```python
from build123d import *

# Parameters (mm, degrees)
RESSALTO_EXTRUS_O1_DEPTH                   = 8
BROCA_DE_ROSQUEAR_PARA_TARRAXA_DE_M6X1_0_D = 5
RESSALTO_EXTRUS_O2_DEPTH                   = 30
ESBO_O6_W                                  = 10
ESBO_O6_H                                  = 40
ESBO_O6_H_2                                = 25
CORTE_EXTRUS_O2_DEPTH                      = 20
ESBO_O14_R                                 = 3
CORTE_EXTRUS_O6_DEPTH                      = 39
ESBO_O15_R                                 = 4.25
CORTE_EXTRUS_O7_DEPTH                      = 40
RESSALTO_EXTRUS_O3_DEPTH                   = 10
ESBO_O17_W                                 = 60
ESBO_O17_H                                 = 9.5
RESSALTO_EXTRUS_O4_DEPTH                   = 30
ESBO_O18_W                                 = 9.5
ESBO_O18_H                                 = 40
RESSALTO_EXTRUS_O5_DEPTH                   = 30
FILETE1_R                                  = 5
ESBO_O19_R                                 = 2.5
CORTE_EXTRUS_O8_DEPTH                      = 10
ESBO_O20_R                                 = 2.5
CORTE_EXTRUS_O9_DEPTH                      = 10


with BuildPart() as part:
    # Esboço1 → Ressalto-extrusão1 (new body)
    with BuildSketch(Plane.XY):
        with BuildLine():
            Line((440, 72.212171493), (380, 72.212171493))
            Line((380, 72.212171493), (380, 132.212171493))
            ThreePointArc((380, 132.212171493), (382.928932188, 139.283239304), (390, 142.212171493))
            Line((390, 142.212171493), (470, 142.212171493))
            Line((470, 142.212171493), (470, 102.212171493))
            Line((470, 102.212171493), (440, 102.212171493))
            Line((440, 102.212171493), (440, 72.212171493))
        make_face()
    extrude(amount=RESSALTO_EXTRUS_O1_DEPTH)

    # Broca de rosquear para tarraxa de M6x1.01 (through all)
    with Locations(Plane.XY.offset(8)):
        with Locations((393, 87.212171493), (427, 87.212171493), (455, 112.212171493), (455, 132.212171493)):
            Hole(BROCA_DE_ROSQUEAR_PARA_TARRAXA_DE_M6X1_0_D / 2)

    # Esboço4 → Ressalto-extrusão2 (add)
    with BuildSketch(Plane(origin=(0, 0, 0), x_dir=(-1, 0, 0), z_dir=(0, 0, -1))):
        with BuildLine():
            Line((-390, 142.212171493), (-440, 142.212171493))
            Line((-440, 142.212171493), (-440, 102.212171493))
            Line((-440, 102.212171493), (-380, 102.212171493))
            Line((-380, 102.212171493), (-380, 132.212171493))
            ThreePointArc((-380, 132.212171493), (-382.928932188, 139.283239304), (-390, 142.212171493))
        make_face()
    extrude(amount=RESSALTO_EXTRUS_O2_DEPTH)

    # Esboço6 → Corte-extrusão2 (cut)
    with BuildSketch(Plane.ZY.offset(-380)):
        with Locations((-22.874860756, 122.212171493)):
            Rectangle(ESBO_O6_W, ESBO_O6_H)
        with Locations((-8.874860756, 129.712171493)):
            Rectangle(ESBO_O6_W, ESBO_O6_H_2)
    extrude(amount=-CORTE_EXTRUS_O2_DEPTH, mode=Mode.SUBTRACT)

    # Esboço14 → Corte-extrusão6 (cut, through all)
    with BuildSketch(Plane(origin=(0, 0, -30), x_dir=(-1, 0, 0), z_dir=(0, 0, -1))):
        with Locations((-390, 129.712171493)):
            Circle(ESBO_O14_R)
        with Locations((-390, 114.712171493)):
            Circle(ESBO_O14_R)
    extrude(amount=-CORTE_EXTRUS_O6_DEPTH, mode=Mode.SUBTRACT)

    # Esboço15 → Corte-extrusão7 (cut)
    with BuildSketch(Plane(origin=(0, 142.212171493, 0), x_dir=(1, 0, 0), z_dir=(0, 1, 0))):
        with Locations((420, 18.90241208)):
            Circle(ESBO_O15_R)
        with Locations((420, 1.90241208)):
            Circle(ESBO_O15_R)
    extrude(amount=-CORTE_EXTRUS_O7_DEPTH, mode=Mode.SUBTRACT)

    # Esboço16 → Ressalto-extrusão3 (add)
    with BuildSketch(Plane(origin=(0, 0, -30), x_dir=(-1, 0, 0), z_dir=(0, 0, -1))):
        with BuildLine():
            Line((-380, 102.212171493), (-440, 102.212171493))
            Line((-440, 102.212171493), (-440, 110.212171493))
            Line((-440, 110.212171493), (-440, 142.212171493))
            Line((-440, 142.212171493), (-432, 142.212171493))
            Line((-432, 142.212171493), (-432, 110.212171493))
            Line((-432, 110.212171493), (-394.815024021, 110.212171493))
            ThreePointArc((-394.815024021, 110.212171493), (-391.180367629, 108.706647521), (-387.545711238, 110.212171493))
            Line((-387.545711238, 110.212171493), (-380, 110.212171493))
            Line((-380, 110.212171493), (-380, 102.212171493))
        make_face()
    extrude(amount=RESSALTO_EXTRUS_O3_DEPTH)

    # Esboço17 → Ressalto-extrusão4 (add, through all)
    with BuildSketch(Plane.XZ.offset(-102.212171493)):
        with Locations((410, -35.25)):
            Rectangle(ESBO_O17_W, ESBO_O17_H)
    extrude(amount=RESSALTO_EXTRUS_O4_DEPTH)

    # Esboço18 → Ressalto-extrusão5 (add, through all)
    with BuildSketch(Plane(origin=(440, 0, 0), x_dir=(0, 0, -1), z_dir=(1, 0, 0))):
        with Locations((35.25, 122.212171493)):
            Rectangle(ESBO_O18_W, ESBO_O18_H)
    extrude(amount=RESSALTO_EXTRUS_O5_DEPTH)

    # Filete1
    filete1_edges = [part.edges().sort_by_distance(p)[0] for p in [
        (432, 110.212171493, -35),
    ]]
    fillet(filete1_edges, radius=FILETE1_R)

    # Esboço19 → Corte-extrusão8 (cut)
    with BuildSketch(Plane.XY.offset(-30.5)):
        with Locations((455, 132.212171493)):
            Circle(ESBO_O19_R)
        with Locations((455, 112.212171493)):
            Circle(ESBO_O19_R)
    extrude(amount=-CORTE_EXTRUS_O8_DEPTH, mode=Mode.SUBTRACT)

    # Esboço20 → Corte-extrusão9 (cut)
    with BuildSketch(Plane.XY.offset(-30.5)):
        with Locations((427, 87.212171493)):
            Circle(ESBO_O20_R)
        with Locations((393, 87.212171493)):
            Circle(ESBO_O20_R)
    extrude(amount=-CORTE_EXTRUS_O9_DEPTH, mode=Mode.SUBTRACT)


solid = part.part
```
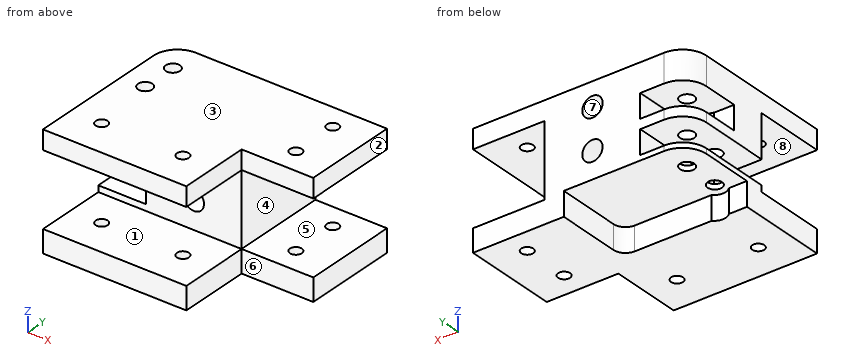
Could you check a few things on this model? Use its own coordinates, in mm. Face numbers are marked on the shaded views. A direction names the side the tool comes from. Give positions to 0.01 mm unless a question says otherwise; leave off trailing zeros. Order: outer loops, then holes, each group sorted by start corner. A loop starts at its lowest first (then second) coordinate and runs counter-clockwise, first axis right, second up.
Q1. Suppose I cut it at C-C, the plane z = -11. Write out the boundary of the cut face in (x, y).
Q2. Suppose I cut it at D-D, the plane x = 455. Write out the boundary of the cut face in (y, z).
Q3. Suppose I cut it at B-B, the plane y = 92.5. Write out the boundary of the cut face in (x, z).
Q4. We'd pull the mould along Z, two halves only. Please class the marked faces 1, 2, 3 and 4: +Z half, -Z half, draft (parallel to the pull), parting line (faces both ways), or undercut.
Q5. If I drill on line 1 along Y through (x, z) = (390, -28.6); line 2 along Z through (x, y) = (464, 104.5); line 3 along Y through (x, z) = (427, 2), over which ranges is the centre line in solid material (lowest first)?
Q6. Suppose I cut it at A-A, the plane x = 420. Write out the boundary of the cut face in (y, z), and give its area (4 significant figures).
Q7. I'm going to push flat-ended pins straight in: P1, Ø16, axis at x = 393.5, y = 122, coming from the -Z side; P2, Ø4, axis at x = 454, z = 5.5, coming from the -Y side; P3, Ø9, axis at y = 93.5, z = 4, coming from the +X side. Where does each tip first touch, or does it pass through?
Q8. For the marked faces 5, 6, 7 and 8, which set-ups out of +Z, -Z, +X, -X, +Y, -Y let a thin tool reach every point of the face, with its end or its side?
Solution:
1. outline: (380, 102.21) - (440, 102.21) - (440, 142.21) - (400, 142.21) - (400, 117.21) - (391.66, 117.21) arc R3 cw (long way) to (388.34, 117.21) - (380, 117.21) - close
2. outline: (102.21, -40) - (109.71, -40) - (109.71, -30.5) - (102.21, -30.5) - close; (102.21, 0) - (109.71, 0) - (109.71, 8) - (102.21, 8) - close; (114.71, -40) - (129.71, -40) - (129.71, -30.5) - (114.71, -30.5) - close; (114.71, 0) - (129.71, 0) - (129.71, 8) - (114.71, 8) - close; (134.71, -40) - (142.21, -40) - (142.21, -30.5) - (134.71, -30.5) - close; (134.71, 0) - (142.21, 0) - (142.21, 8) - (134.71, 8) - close
3. outline: (380, -40) - (440, -40) - (440, -30.5) - (380, -30.5) - close; (380, 0) - (440, 0) - (440, 8) - (380, 8) - close
4. face 1: undercut
4. face 2: draft
4. face 3: +Z half
4. face 4: undercut
5. line 1: y = 102.21 to 111.71, 117.71 to 126.71, 132.71 to 142.21
5. line 2: z = -40 to -30.5, 0 to 8
5. line 3: y = 72.21 to 84.71, 89.71 to 142.21
6. outline: (72.21, -40) - (110.21, -40) - (110.21, -30) - (142.21, -30) - (142.21, -23.15) - (102.21, -23.15) - (102.21, -30.5) - (72.21, -30.5) - close; (72.21, 0) - (102.21, 0) - (102.21, 2.35) - (142.21, 2.35) - (142.21, 8) - (72.21, 8) - close; (102.21, -14.65) - (142.21, -14.65) - (142.21, -6.15) - (102.21, -6.15) - close
6. area: 1,445 mm2
7. P1: stops at z = -30
7. P2: stops at y = 102.21
7. P3: stops at x = 440
8. face 5: +X, +Y, -Y
8. face 6: +Z, -Z, +X, -Y
8. face 7: +Y
8. face 8: +X, -X, -Y
